Part model, mm, in its own coordinate system. Face numbers are marked on the shaded views. A direction names the side the tool comes from. Coordinates: 2 decimals unless noted, no trailing zeros. Loops run counter-clockwise (first coordinate to the right, second up) from the corner with the lowest first, then second, coordinate; pieces in that order, holes last. Notation, with made-up numbers: (12, -4) -> (67, -4) arc R20 ccw to (67, 1) -> close; hole circle Ø3 at (25, -34.75). An arc over 180 degrees is marked (long way). Use one line per item in the form item = value. Start each with the question number.
(1) Band-saw the part on A-A on x = 8. Give the cut face in (y, z), then the cut area to 3 significant figures.
(2) 3-axis set-ups, long thin cutter, end or side, ignore diameter. For the marked faces 1, 2 and 3: which of +Z, -Z, +X, -X, +Y, -Y reach the whole face in a straight line?
(3) Pin check, flat tips, straight feed: P1, Ø1.5, axis at y = -8, z = 0.5, coming from the +X side; P2, Ø1, axis at x = 5.5, z = 1, coming from the +Y side; P3, Ø1.5, axis at x = -12.5, z = 0, coming from the +Y side. Stop position of each tip, or through.
(4) Drill centre lines: L1, parallel to Y at x = 0, z = 0.4; L2, parallel to X at y = 4, z = 1.25; L3, parallel to Y at x = 11, z = 1.05. Where is each one in solid material? Low to high. Write a range as [from, to].
(5) Mould opens along X. For the marked faces 4, 5 and 6 say: +X half, -X half, draft (parallel to the pull), parting line (faces both ways), or undercut.
(6) Band-saw the part on C-C on y = 8. Give the cut face in (x, z), then the cut area to 3 significant figures.
(7) Band-saw the part on D-D on x = 0. Give the cut face in (y, z), then the cut area to 3 significant figures.
(8) Band-saw the part on B-B on z = -0.45. Give the cut face in (x, y).
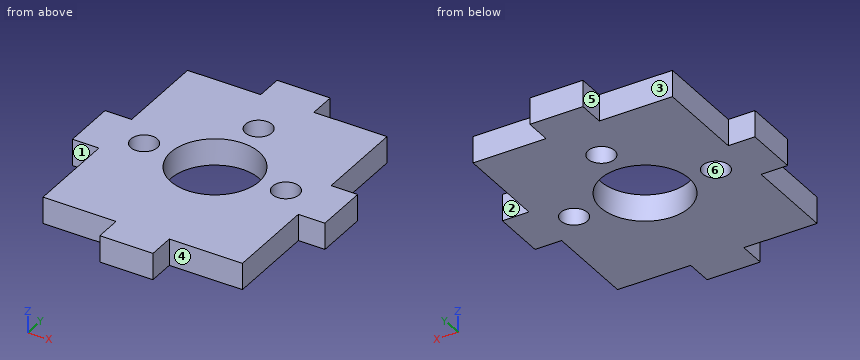
```python
from build123d import *

# Parameters (mm, degrees)
SKETCH_W     = 22.5
SKETCH_H     = 26.5
SKETCH_R     = 5
SKETCH_R_2   = 1.5
PAD_DEPTH    = 1.5
SKETCH017_W  = 6
SKETCH017_H  = 3
PAD005_DEPTH = 3
SKETCH018_W  = 3
SKETCH018_H  = 6
PAD006_DEPTH = 3


with BuildPart() as part:
    # Sketch → Pad (new body, symmetric)
    with BuildSketch(Plane.XY):
        Rectangle(SKETCH_W, SKETCH_H)
        Circle(SKETCH_R, mode=Mode.SUBTRACT)
        with Locations((0, 8)):
            Circle(SKETCH_R_2, mode=Mode.SUBTRACT)
        with Locations((8, 0)):
            Circle(SKETCH_R_2, mode=Mode.SUBTRACT)
        with Locations((-8, 0)):
            Circle(SKETCH_R_2, mode=Mode.SUBTRACT)
    extrude(amount=PAD_DEPTH, both=True)

    # Sketch017 (on Face10 of Pad) → Pad005 (join)
    with BuildSketch(Plane.XY.offset(1.5)):
        with Locations((0, 14.75)):
            Rectangle(SKETCH017_W, SKETCH017_H)
        with Locations((0, -14.75)):
            Rectangle(SKETCH017_W, SKETCH017_H)
    extrude(amount=-PAD005_DEPTH)

    # Sketch018 (on Face18 of Pad005) → Pad006 (join)
    with BuildSketch(Plane.XY.offset(1.5)):
        with Locations((-12.75, 0)):
            Rectangle(SKETCH018_W, SKETCH018_H)
        with Locations((12.75, 0)):
            Rectangle(SKETCH018_W, SKETCH018_H)
    extrude(amount=-PAD006_DEPTH)


solid = part.part
```
A:
q1.outline = (-13.25, -1.5) -> (-1.5, -1.5) -> (-1.5, 1.5) -> (-13.25, 1.5) -> close; (1.5, -1.5) -> (13.25, -1.5) -> (13.25, 1.5) -> (1.5, 1.5) -> close
q1.area = 70.5 mm²
q2.face_1 = +Z, -Z, -X, -Y
q2.face_2 = +Z, -Z, +X, +Y
q2.face_3 = +Z, -Z, -X, +Y
q3.P1 = 11.25
q3.P2 = 13.25
q3.P3 = 3
q4.L1 = [-16.25, -5], [5, 6.5], [9.5, 16.25]
q4.L2 = [-11.25, -3], [3, 11.25]
q4.L3 = [-13.25, 13.25]
q5.face_4 = draft
q5.face_5 = -X half
q5.face_6 = undercut
q6.outline = (-11.25, -1.5) -> (-1.5, -1.5) -> (-1.5, 1.5) -> (-11.25, 1.5) -> close; (1.5, -1.5) -> (11.25, -1.5) -> (11.25, 1.5) -> (1.5, 1.5) -> close
q6.area = 58.5 mm²
q7.outline = (-16.25, -1.5) -> (-5, -1.5) -> (-5, 1.5) -> (-16.25, 1.5) -> close; (5, -1.5) -> (6.5, -1.5) -> (6.5, 1.5) -> (5, 1.5) -> close; (9.5, -1.5) -> (16.25, -1.5) -> (16.25, 1.5) -> (9.5, 1.5) -> close
q7.area = 58.5 mm²
q8.outline = (-14.25, -3) -> (-11.25, -3) -> (-11.25, -13.25) -> (-3, -13.25) -> (-3, -16.25) -> (3, -16.25) -> (3, -13.25) -> (11.25, -13.25) -> (11.25, -3) -> (14.25, -3) -> (14.25, 3) -> (11.25, 3) -> (11.25, 13.25) -> (3, 13.25) -> (3, 16.25) -> (-3, 16.25) -> (-3, 13.25) -> (-11.25, 13.25) -> (-11.25, 3) -> (-14.25, 3) -> close; hole circle Ø3 at (-8, 0); hole circle Ø10 at (0, 0); hole circle Ø3 at (0, 8); hole circle Ø3 at (8, 0)
